Part model, mm, in its own coordinate system. Face numbers are marked on the shaded views. Give positions to 0.01 mm unless a question says otherwise; leave off trailing zeros. Order: outer loops, then holes, each group sorted by start corner. A loop starts at its lowest first (then second) coordinate and runs counter-clockwise, first axis right, second up. Notation, with made-up numbers: (23, -10) -> (52, -10) arc R31 ccw to (52, 22) -> close; hole circle Ø11 at (27, 6.25). An arc over 180 degrees is marked (long way). Write item = value, one per line. Start each with the question number.
(1) Saw through at B-B, the plane z = 0. List the corners of the cut face in (x, y).
(2) Two-plate mould, pull along X, no slides. Class the marked faces 1, 2 and 3: pulls with the +X half, pulls with the -X half, needs draft (parallel to the pull), parting line crosses it, or undercut.
(3) Saw through at A-A, the plane x = 0. List the corners of the cut face in (y, z).
(4) Saw through at D-D, the plane y = 68.5. List the corners of the cut face in (x, z), then the cut area to 3 significant figures.
(5) Flat gauge pins, fed straight in: pin 1 (6 mm diameter, centred on x = -33.5, y = 37, fed in from -Z); pin 2 (1.5 mm diameter, centred on y = 56.5, z = -23, fed in from -X); pin 3 (2 mm diameter, centred on x = 8.5, z = 4.5, fed in from +Y). Where does each tip first touch, or does it go through?
(6) Probe line 1 along X through (y, z) = (11, 11); line 2 along X through (y, z) = (97, -13); line 3 along Y through (x, z) = (28, 6). List the from-to ranges inside material, lowest first. Write a range as from..to.
(7) Saw through at C-C, the plane y = 15.5. List the corners of the cut face in (x, z).
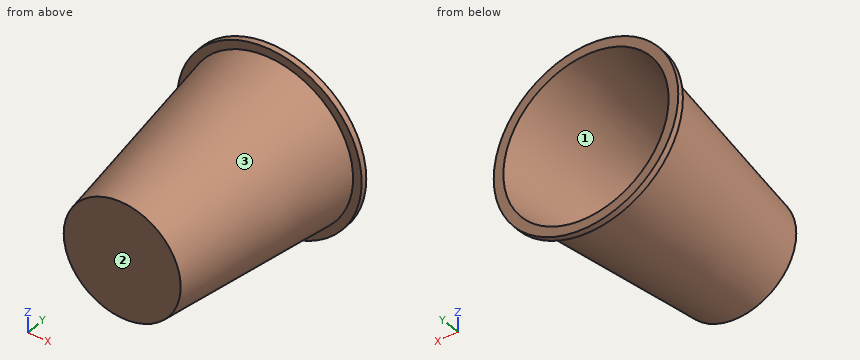
from build123d import *

# Parameters (mm, degrees)
COQUE1_T           = -1
ESQUISSE2_R        = 49.69
ESQUISSE2_R_2      = 44.491785277
BOSS_EXTRU_1_DEPTH = 3.3


with BuildPart() as part:
    # Esquisse1 → Révolution1 (revolve)
    with BuildSketch(Plane.XY, mode=Mode.PRIVATE) as r_volution1_sk:
        Polygon((0, 0), (31.5, 0), (45.5, 109), (0, 109), align=None)
    revolve(r_volution1_sk.sketch.rotate(Axis((0, 109, 0), (0, -1, 0)), 180), axis=Axis((0, 109, 0), (0, -1, 0)))

    # Coque1
    coque1_openings = [part.faces().sort_by_distance(p)[0] for p in [
        (0, 109, 0),
    ]]
    offset(amount=COQUE1_T, openings=coque1_openings, kind=Kind.INTERSECTION)

    # Esquisse2 → Boss.-Extru.1 (add)
    with BuildSketch(Plane(origin=(0, 109, 0), x_dir=(1, 0, 0), z_dir=(0, 1, 0))):
        with Locations(Location((0, 0, 0), (0, 0, 180))):
            Circle(ESQUISSE2_R)
        Circle(ESQUISSE2_R_2, mode=Mode.SUBTRACT)
    extrude(amount=-BOSS_EXTRU_1_DEPTH)


solid = part.part
Results list:
q1.outline = (-49.69, 105.7) -> (-45.08, 105.7) -> (-31.5, 0) -> (31.5, 0) -> (45.08, 105.7) -> (49.69, 105.7) -> (49.69, 109) -> (44.49, 109) -> (30.62, 1) -> (-30.62, 1) -> (-44.49, 109) -> (-49.69, 109) -> close
q2.face_1 = undercut
q2.face_2 = needs draft
q2.face_3 = parting line crosses it
q3.outline = (0, -31.5) -> (105.7, -45.08) -> (105.7, -49.69) -> (109, -49.69) -> (109, -44.49) -> (1, -30.62) -> (1, 30.62) -> (109, 44.49) -> (109, 49.69) -> (105.7, 49.69) -> (105.7, 45.08) -> (0, 31.5) -> close
q4.outline = circle Ø80.6 at (0, 0); hole circle Ø78.58 at (0, 0)
q4.area = 252 mm^2
q5.pin_1 = -19.65
q5.pin_2 = -31.75
q5.pin_3 = 1
q6.line_1 = -31.02..-29.95, 29.95..31.02
q6.line_2 = -41.99..-40.94, 40.94..41.99
q6.line_3 = 0..1
q7.outline = circle Ø66.98 at (0, 0); hole circle Ø64.97 at (0, 0)
